Verification items for this drawing (mm, ordinates from the low corner). A direction names the side the tool comes from. Give positions to 0.01 mm unless a question says otherwise; leave off trailing zeros. Write each loop counter-clockwise with the first axis right and the second up, starting at its lowest first coordinate (ties: lowest second). Pieces come first, ordered by that corner, then holes. Notation, with made-up numbers: (37.25, -30) -> (71.25, -30) arc R25 ccw to (71.25, 3) -> close; hole circle Ø6 at (86, 75.5). An arc over 180 degrees is marked (long way). Use one line per item in the form item = value. Start each with the question number.
(1) Scan lines: L1, parallel to X at y = 15.3, z = 52; L2, parallel to Y at x = 3, z = 44.5; L3, parallel to Z at x = 11, y = 46. Record each from-to range of solid material in increasing order.
(2) Depth check by flat-ended pin: pin 1 Ø2.5 at (y, z) = (37, 2) entering from -X; pin 2 Ø10 at (x, z) = (22.5, 50.5) entering from +Y; pin 3 Ø3.5 at (x, z) = (11.05, 52) entering from -Y. Enter the tip coordinate at first touch or a pass-through.
(3) Release check for a two-part mould opening along X. For the marked faces 4, 5 and 6 record: pulls with the +X half, pulls with the -X half, needs draft (parallel to the pull), parting line crosses it, or undercut.
(4) Section check B-B, the plane y = 10. Record the cut outline in (x, z), plus the area to 3 significant figures.
(5) Set-up check for the marked faces 1, 2 and 3: record each of +Z, -Z, +X, -X, +Y, -Y from which the full face is reachable in a straight line by a thin tool's end or side.
(6) Section check A-A, the plane z = 4. State how many separate pieces and enclosed holes the cut face has, plus the area to 3 significant figures.
(7) Section check C-C, the plane z = 31.5. Record the cut outline in (x, y).
(8) Section check D-D, the plane x = 29. Record the cut outline in (y, z).
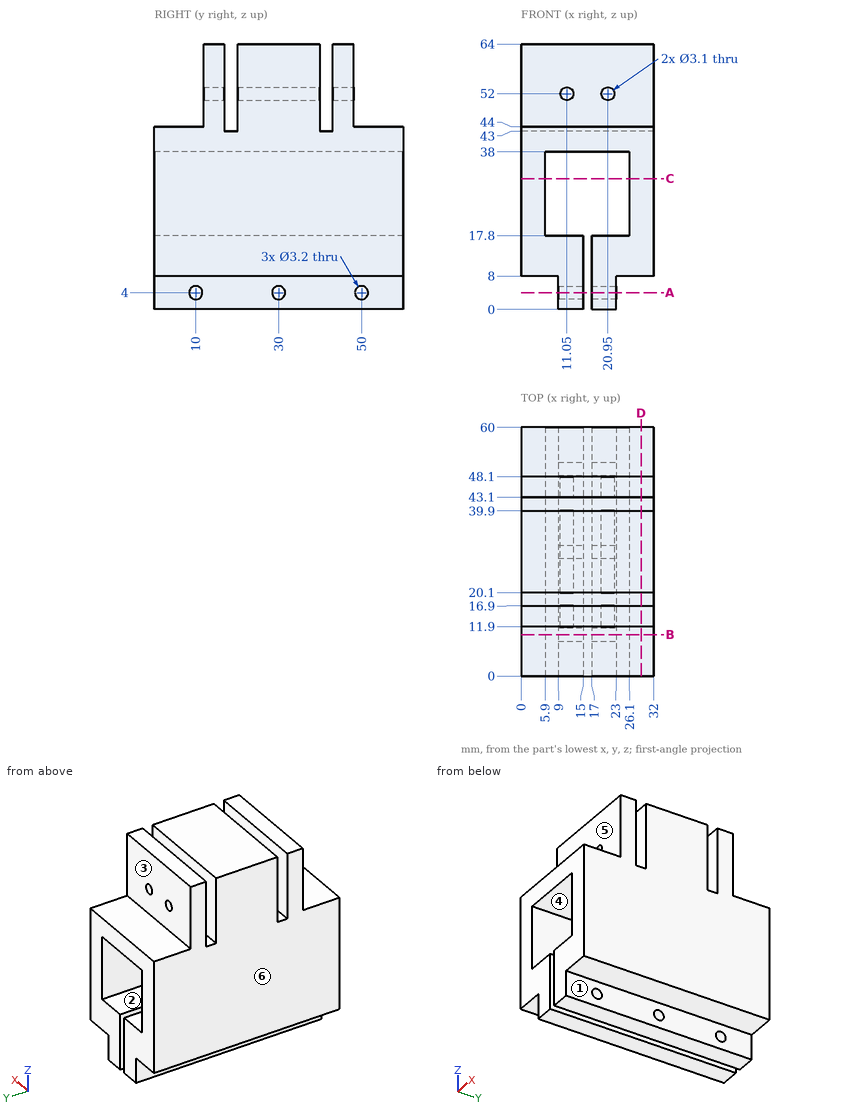
Completed:
q1.L1 = 0 to 9.5, 12.6 to 19.4, 22.5 to 32
q1.L2 = 11.9 to 16.9, 20.1 to 39.9, 43.1 to 48.1
q1.L3 = 0 to 17.8, 38 to 50.45, 53.55 to 64
q2.pin_1 = 9
q2.pin_2 = 48.1
q2.pin_3 = 11.9
q3.face_4 = undercut
q3.face_5 = needs draft
q3.face_6 = pulls with the -X half
q4.outline = (0, 8) -> (9, 8) -> (9, 5.6) -> (15, 5.6) -> (15, 17.8) -> (5.9, 17.8) -> (5.9, 38) -> (26.1, 38) -> (26.1, 17.8) -> (17, 17.8) -> (17, 5.6) -> (23, 5.6) -> (23, 8) -> (32, 8) -> (32, 44) -> (0, 44) -> close; (9, 0) -> (15, 0) -> (15, 2.4) -> (9, 2.4) -> close; (17, 0) -> (23, 0) -> (23, 2.4) -> (17, 2.4) -> close
q4.area = 782 mm²
q5.face_1 = -Z, +X, +Y, -Y
q5.face_2 = +Y, -Y
q5.face_3 = +Z, +X, -X, +Y
q6.separate_pieces = 8
q6.enclosed_holes = 0
q6.area = 605 mm²
q7.outline = (0, 0) -> (5.9, 0) -> (5.9, 60) -> (0, 60) -> close; (26.1, 0) -> (32, 0) -> (32, 60) -> (26.1, 60) -> close
q8.outline = (0, 8) -> (60, 8) -> (60, 44) -> (48.1, 44) -> (48.1, 64) -> (43.1, 64) -> (43.1, 43) -> (39.9, 43) -> (39.9, 64) -> (20.1, 64) -> (20.1, 43) -> (16.9, 43) -> (16.9, 64) -> (11.9, 64) -> (11.9, 44) -> (0, 44) -> close
